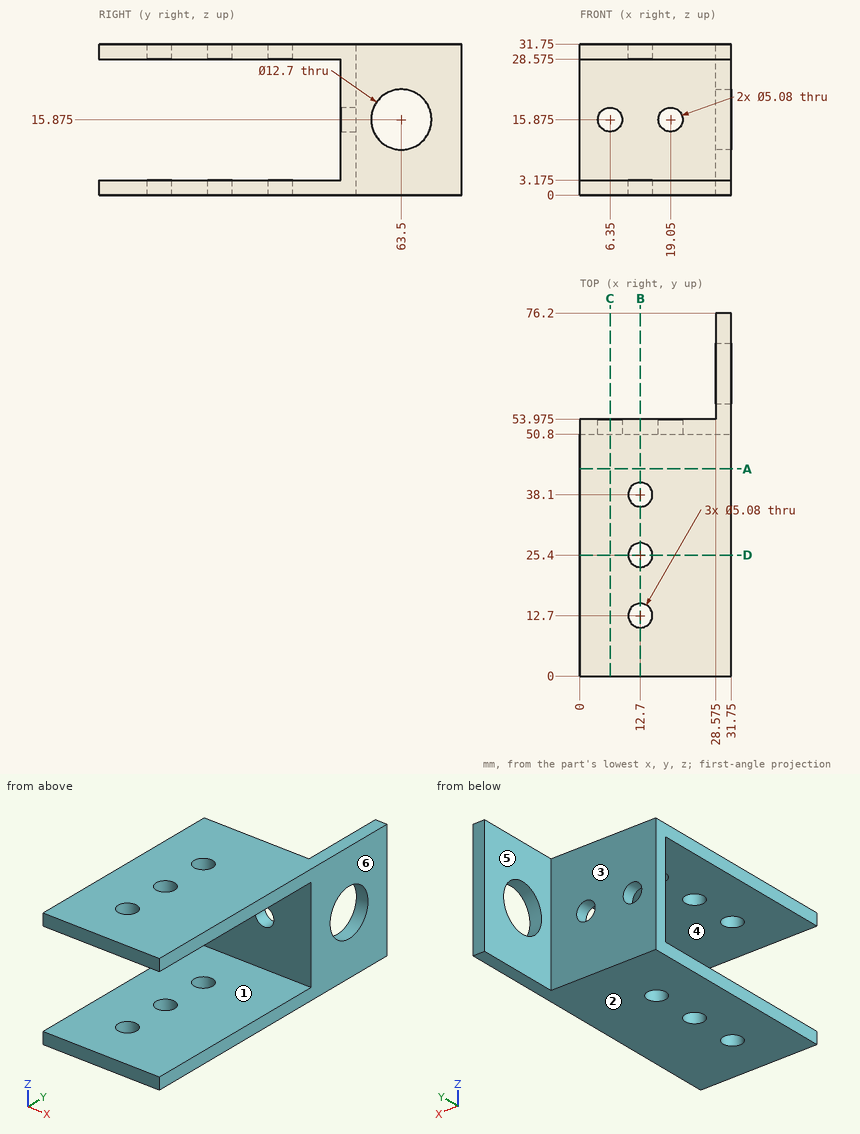
The figure shows three views and two pictorial views of one solid part (mm, origin at its lowest corner). Answer the questions. A direction names the side the tool comes from. Give positions to 0.01 mm unless a question says otherwise; leave off trailing zeros. Order: outer loops, then holes, each group sorted by start corner. A loop starts at its lowest first (then second) coordinate and runs counter-clockwise, first axis right, second up. Notation, with made-up numbers: (60, 82.25) -> (91, 82.25) arc R18 cw to (91, 88.25) -> close; hole circle Ø4 at (26, -18). An arc over 180 degrees is marked (long way). Answer as a JSON object with one key per item and string values. Group by question number.
Item 1: The part is cut by section C-C on x = 6.35. Write down the section's boundary in (y, z) (3 decimals), and give its area (3 significant figures).
Item 2: Determine the mould class of the marked faces 1, 2 and 3 for opening direction Z: pulls with the +Z half, pulls with the -Z half, needs draft (parallel to the pull), parting line crosses it, or undercut.
Item 3: The part is cut by section A-A on y = 43.5. Write down the section's boundary in (x, z) (3 decimals).
Item 4: Consider L1, parallel to Y at x = 12.7, z = 30.9 (3 decimals); L2, parallel to Z at x = 23.5, y = 28 (3 decimals); L3, parallel to Y at x = 12, z = 29 (3 decimals). Determine where each line is inside the solid, lowest interval first. Write a range as from..to.
Item 5: Flat-ended cylindrical pins translate along their axes: pin 1 (4 mm diameter, centred on x = 12.7, y = 38.1, fed in from -Z); pin 2 (6.5 mm diameter, centred on x = 6.35, z = 15.875, fed in from +Y) (3 decimals); pin 3 (11 mm diameter, centred on y = 66, z = 12, fed in from -X) (3 decimals); pin 4 (7.5 mm diameter, centred on x = 9, z = 20.5, fed in from -Y). Find the tip coordinate at first contact, or state that the pin passes through.
Item 6: The part is cut by section D-D on y = 25.4. Write down the section's boundary in (x, z) (3 decimals).
Item 7: The part is cut by section B-B on x = 12.7. Give the number of separate pieces and of enclosed holes in the cut face, and give its area (3 significant figures).
Item 8: A tool of negligible diameter and unlimited length cuts with its end or side. For the marked faces 4, 5 and 6, from which of +Z, -Z, +X, -X, +Y, -Y can it reach the whole face along a straight path? Write none if from no direction.
Result set:
{
 "1": {"outline": "(0, 0) -> (53.975, 0) -> (53.975, 13.335) -> (50.8, 13.335) -> (50.8, 3.175) -> (0, 3.175) -> close; (0, 28.575) -> (50.8, 28.575) -> (50.8, 18.415) -> (53.975, 18.415) -> (53.975, 31.75) -> (0, 31.75) -> close", "area": "407 mm²"},
 "2": {"face 1": "undercut", "face 2": "pulls with the -Z half", "face 3": "needs draft"},
 "3": {"outline": "(0, 0) -> (31.75, 0) -> (31.75, 3.175) -> (0, 3.175) -> close; (0, 28.575) -> (31.75, 28.575) -> (31.75, 31.75) -> (0, 31.75) -> close"},
 "4": {"L1": "0..10.16, 15.24..22.86, 27.94..35.56, 40.64..53.975", "L2": "0..3.175, 28.575..31.75", "L3": "0..10.258, 15.142..22.958, 27.842..35.658, 40.542..53.975"},
 "5": {"pin 1": "through", "pin 2": "y = 53.975", "pin 3": "x = 28.575", "pin 4": "y = 50.8"},
 "6": {"outline": "(0, 0) -> (10.16, 0) -> (10.16, 3.175) -> (0, 3.175) -> close; (0, 28.575) -> (10.16, 28.575) -> (10.16, 31.75) -> (0, 31.75) -> close; (15.24, 0) -> (31.75, 0) -> (31.75, 3.175) -> (15.24, 3.175) -> close; (15.24, 28.575) -> (31.75, 28.575) -> (31.75, 31.75) -> (15.24, 31.75) -> close"},
 "7": {"separate pieces": "7", "enclosed holes": "0", "area": "327 mm²"},
 "8": {"face 4": "+X, -X, -Y", "face 5": "+Z, -Z, -X, +Y", "face 6": "+Z, -Z, +X, +Y, -Y"}
}
